For this review, use the dimensioned drawing (mm, ordinates from the lowest corner) and the shaded views. A direction names the side the tool comes from. Round coordinates to 2 decimals unless told otherwise and drop trailing zeros. Loops run counter-clockwise (first coordinate to the right, second up) from the corner with the lowest first, then second, coordinate; pieces in that order, holes last. Notation, with made-up numbers: (-29.5, -36.75) -> (-23.5, -36.75) arc R19 cw to (-23.5, -9.75) -> close; hole circle Ø7 at (82, 71). An arc over 180 degrees is marked (long way). Write each question's results on one line, items separated by ' | '. Start each with the question number.
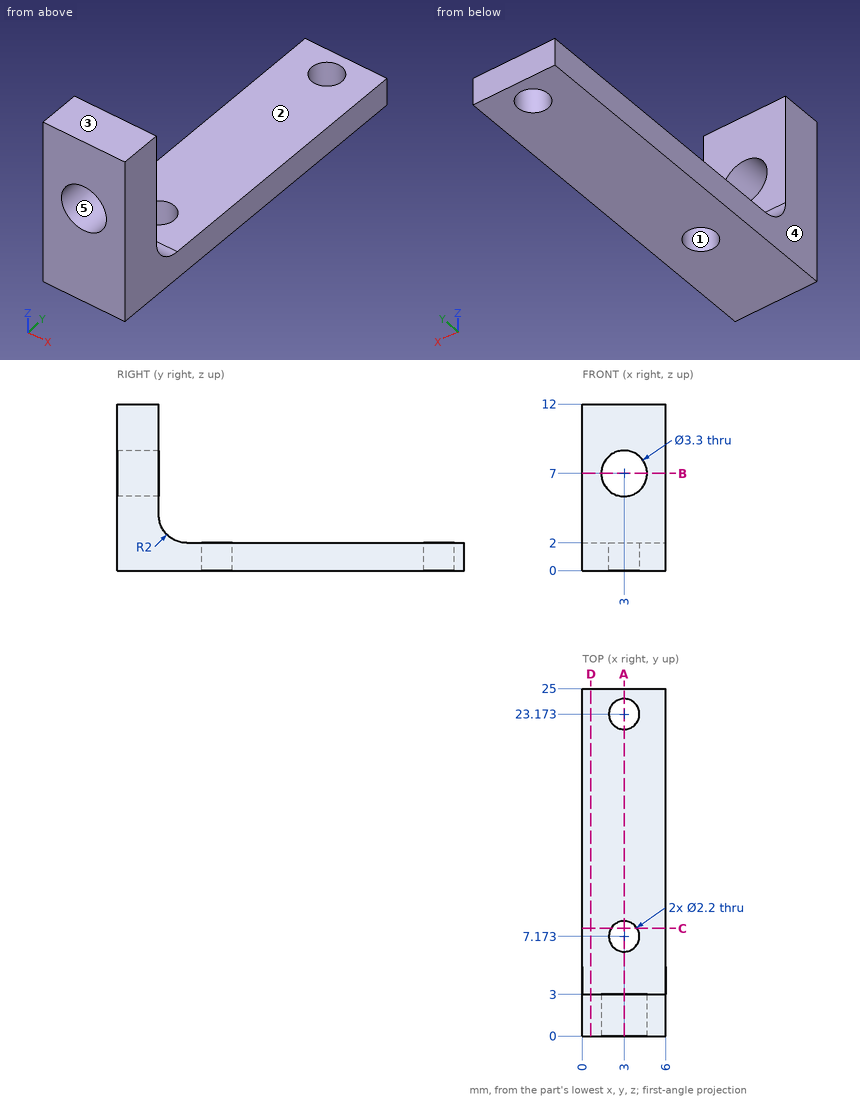
1) Take a section at C-C (y = 7.75). Write out the cut boundary in (x, z).
2) Take a section at D-D (x = 0.6). Write out the cut boundary in (y, z).
3) Take a section at A-A (x = 3). Write out the cut boundary in (y, z).
4) The part is to be moulded in two halves that separate along Z. For the marked faces 3, 4 and 5, say which applies: +Z half, -Z half, draft (parallel to the pull), parting line (faces both ways), or undercut.
5) For the marked faces 1 and 2, list the 3-axis set-ups (+Z, -Z, +X, -X, +Y, -Y) from which the entire face can be reached by the end or side of a thin tool; tool diameter is ignored.
6) Insertion check: pin 1 (3 mm diameter, centred on x = 3, y = 15.5, fed in from +Z); pin 2 (3 mm diameter, centred on x = 2, z = 7, fed in from +Y). Each pin has a flat end and moves straight along its axis. Give the tip position at first contact, or say it passes through.
7) Take a section at B-B (z = 7). Write out the cut boundary in (x, y).
8) To check wall thickness, follow line 1 (Y direction, x = 3, z = 1.2); line 2 (Z direction, x = 3, y = 1.25); line 3 (Z direction, x = 2.7, y = 19.25). State the ranges of each line that lie inside material, in increasing order. Write a range as from..to.
Geometry check:
1) outline: (0, 0) -> (2.06, 0) -> (2.06, 2) -> (0, 2) -> close; (3.94, 0) -> (6, 0) -> (6, 2) -> (3.94, 2) -> close
2) outline: (0, 0) -> (25, 0) -> (25, 2) -> (5, 2) arc R2 cw to (3, 4) -> (3, 12) -> (0, 12) -> close
3) outline: (0, 0) -> (6.07, 0) -> (6.07, 2) -> (5, 2) arc R2 cw to (3, 4) -> (3, 5.35) -> (0, 5.35) -> close; (0, 8.65) -> (3, 8.65) -> (3, 12) -> (0, 12) -> close; (8.27, 0) -> (22.07, 0) -> (22.07, 2) -> (8.27, 2) -> close; (24.27, 0) -> (25, 0) -> (25, 2) -> (24.27, 2) -> close
4) face 3: +Z half | face 4: draft | face 5: undercut
5) face 1: +Z, -Z | face 2: +Z, +X, -X, +Y
6) pin 1: stops at z = 2 | pin 2: stops at y = 3
7) outline: (0, 0) -> (1.35, 0) -> (1.35, 3) -> (0, 3) -> close; (4.65, 0) -> (6, 0) -> (6, 3) -> (4.65, 3) -> close
8) line 1: y = 0..6.07, 8.27..22.07, 24.27..25 | line 2: z = 0..5.35, 8.65..12 | line 3: z = 0..2
